The model under review builds one solid part; all positions refer to its coordinate system, in mm. A direction names the side the tool comes from. Round coordinates to 2 decimals unless told otherwise and drop trailing zeros. Order: outer loops, then holes, each group sorted by start corner. A loop starts at its lowest first (then second) coordinate and runs counter-clockwise, first axis right, second up. Notation, with made-up numbers: M 48,-25 L 71,-25 A19 ccw 71,4 Z; hole C 33.25,87.5 d8. An arc over 180 degrees is marked long. Answer as a JSON object with one key per item and string values. Group by question number.
1. Add section C-C on z = 10. State the section outline as (x, y) points, and give its area (3 significant figures).
2. Mouldability with a two-part tool opening along Y and no side actions: class faces 1 (the face through (0.748, 0.976, 5.916)), 2 (the face through (-2.5, 0, 10)), 3 (the face through (-3, 0, 6)) as released by +Y, released by -Y, zero draft, split by the parting line, or undercut.
3. Machinability: for faces 4 (the face through (2.5, 0, 10)), 5 (the face through (1, -1, 12)), which of the approach directions +Z, -Z, +X, -X, +Y, -Y give a long, thin tool a straight path to every point of the face, cutting with its end or side? Answer none if there is none.
4. Add section B-B on y = -0.3. State the section outline as (x, z) points, and give its area (3 significant figures).
5. Add section D-D on y = 1.4. State the section outline as (x, z) points, and give its area (3 significant figures).
6. Clearance check with flat-ended pins moving along their axes: P1, Ø3.5, axis at y = -0.5, z = 10, coming from the +X side; P2, Ø1, axis at y = -0.5, z = 10, coming from the -X side; P3, Ø2, axis at x = 0, y = 0, coming from the +Z side. State where each tip first meets the part, or that it passes through.
7. Add section A-A on x = 0. State the section outline as (y, z) points.
8. To check wall thickness, follow probe 1 along X at (y, z) = (0, 3.75); probe 2 along X at (y, z) = (0, 9). State the ranges of each line that lie inside material, in increasing order. Write a range as [from, to].
Autodesk Inventor part; units mm, degrees
ref_plane "YZ Plane" through (0, 0, 0) normal (1, 0, 0) x (0, 1, 0)
ref_plane "XZ Plane" through (0, 0, 0) normal (0, 1, 0) x (-1, 0, 0)
ref_plane "XY Plane" through (0, 0, 0) normal (0, 0, 1) x (1, 0, 0)
sketch "Sketch1" plane through (0, 0, 0) normal (0, 0, 1) x (1, 0, 0)
  circle A0 centre (0, 0) radius 3
  dimension "d0" = 6
extrude "Extrusion1" add sketch "Sketch1" along normal blind 12
sketch "Sketch2" plane through (0, 0, 12) normal (0, 0, 1) x (1, 0, 0)
  point P0 (0, 0)
  point P1 (0, 0)
hole "Hole1" at (0, 0, 12) direction (0, 0, -1) diameter 2.459 end through all
sketch "Sketch3" plane through (0, 0, 0) normal (0, 1, 0) x (-1, 0, 0)
  line L0 (3, 0) -> (3, 12)
  line L1 (3, 12) -> (2.5, 12)
  line L2 (2.5, 12) -> (2.5, 8)
  line L3 (2.5, 8) -> (3, 8)
  line L4 (3, 8) -> (3, 12)
  line L5 (3, 12) -> (-3, 12)
  line L6 (-3, 12) -> (-2.5, 12)
  line L7 (-2.5, 12) -> (-2.5, 8)
  line L8 (-2.5, 8) -> (-3, 8)
  line L9 (-3, 8) -> (-3, 12)
  point P0 (0, 0)
  dimension "d10" = 0.5
  dimension "d11" = 5
  dimension "d12" = 0.5
  dimension "d13" = 4
extrude "Extrusion2" cut sketch "Sketch3" along normal through all both and the other way through all
equation "\"d10\" = d12"
properties part number "Pancake_Lever Weight 2" material "Aluminum 6061"
Recorded:
{
 "1": {"outline": "M -2.5,-1.66 A3 ccw 2.5,-1.66 L 2.5,1.66 A3 ccw -2.5,1.66 Z; hole C 0,0 d2.46", "area": "21.3 mm²"},
 "2": {"face 1": "undercut", "face 2": "zero draft", "face 3": "split by the parting line"},
 "3": {"face 4": "+Z, +X, +Y, -Y", "face 5": "+Z, +X, -X, +Y, -Y"},
 "4": {"outline": "M -2.98,0 L -1.19,0 L -1.19,12 L -2.5,12 L -2.5,8 L -2.98,8 Z; M 1.19,0 L 2.98,0 L 2.98,8 L 2.5,8 L 2.5,12 L 1.19,12 Z", "area": "39.1 mm²"},
 "5": {"outline": "M -2.65,0 L 2.65,0 L 2.65,8 L 2.5,8 L 2.5,12 L -2.5,12 L -2.5,8 L -2.65,8 Z", "area": "62.5 mm²"},
 "6": {"P1": "stops at x = 2.5", "P2": "stops at x = -2.5", "P3": "passes through"},
 "7": {"outline": "M -3,0 L -1.23,0 L -1.23,12 L -3,12 Z; M 1.23,0 L 3,0 L 3,12 L 1.23,12 Z"},
 "8": {"probe 1": "x = [-3, -1.23], [1.23, 3]", "probe 2": "x = [-2.5, -1.23], [1.23, 2.5]"}
}
